Here's how the part is built. I have some questions about the finished solid (model axes, mm). A direction names the side the tool comes from. Round coordinates to 2 decimals unless told otherwise and drop trailing zeros. Write each loop counter-clockwise with the first axis right and the second up, starting at its lowest first coordinate (ties: lowest second). Pieces come first, ordered by that corner, then holes. Notation, with made-up numbers: (23.25, 12.25) -> (52.25, 12.25) arc R18 ccw to (52.25, 42.25) -> close; hole circle Ø7 at (-19, -6). An arc over 180 degrees is marked (long way). Put each result on its own line as item: value. Start each with the question number.
1) I want a section at A-A, the plane y = -15. List the corners of the cut face in (x, z) for me, then the cut area to 3 significant figures.
2) Which directions (+Z, -Z, +X, -X, +Y, -Y) give clear straight access to the entire face, cutting with the end or side of a thin tool? Please do faces 1 (the flat face through (-27.5, -15, -2)), 2 (the flat face through (-24, -15, -5)), 3 (the flat face through (24, -15, -5)).
3) We'd pull the mould along X, two halves only. Please class faces 4 (the flat face through (-23, -15, 0)), 5 (the cylindrical face through (0, -15, -15)), 6 (the cylindrical face through (-17.5, -14.9, -2.5)): released by +X, released by -X, zero draft, split by the parting line, or undercut.
4) Will these pins go through, and if not, where does the flat tip stop? P1, Ø6, axis at x = -8, z = -2, coming from the -Y side; P2, Ø4, axis at x = 19.5, y = -19, coming from the -Z side; P3, Ø4, axis at x = 8, y = -5, coming from the -Z side; P4, Ø1.5, axis at y = -21.5, z = -12.5, coming from the -X side.
5) If I drill on line 1 along Y through (x, z) = (-20, -3.65); line 2 along X through (y, z) = (-17, -4.25); line 3 along X through (y, z) = (-10.25, -4), over which ranges is the centre line in solid material (lowest first)? Write a range as [from, to].
6) I want a section at B-B, the plane x = 20. List the corners of the cut face in (y, z) for me, then the cut area to 3 significant figures.
7) I want a section at D-D, the plane z = -11.5. List the corners of the cut face in (x, y) for me, then the cut area to 3 significant figures.
8) I want a section at C-C, the plane z = -3.25. List the corners of the cut face in (x, y) for me, then the cut area to 3 significant figures.
from build123d import *

# Parameters (mm, degrees)
F1_DEPTH = 30
F3_D     = 5


with BuildPart() as f1:
    # F0 (on Front) → F1 (new body)
    with BuildSketch(Plane.XZ):
        with BuildLine():
            ThreePointArc((-14.1421356237, -5), (-14.7839783948, -2.5365296809), (-15, 0))
            Line((-15, 0), (-27.5, 0))
            Line((-27.5, 0), (-27.5, -5))
            Line((-27.5, -5), (-14.1421356237, -5))
        make_face()
        with BuildLine():
            ThreePointArc((-11.4564392374, -5), (-12.2363289116, -2.5538705461), (-12.5, 0))
            Line((-12.5, 0), (-15, 0))
            ThreePointArc((-15, 0), (-14.7839783948, -2.5365296809), (-14.1421356237, -5))
            Line((-14.1421356237, -5), (-11.4564392374, -5))
        make_face()
        with BuildLine():
            ThreePointArc((11.4564392374, -5), (0, -12.5), (-11.4564392374, -5))
            Line((-11.4564392374, -5), (-14.1421356237, -5))
            ThreePointArc((-14.1421356237, -5), (0, -15), (14.1421356237, -5))
            Line((14.1421356237, -5), (11.4564392374, -5))
        make_face()
        with BuildLine():
            ThreePointArc((12.5, 0), (12.2363289116, -2.5538705461), (11.4564392374, -5))
            Line((11.4564392374, -5), (14.1421356237, -5))
            ThreePointArc((14.1421356237, -5), (14.7839783948, -2.5365296809), (15, 0))
            Line((15, 0), (12.5, 0))
        make_face()
        with BuildLine():
            ThreePointArc((15, 0), (14.7839783948, -2.5365296809), (14.1421356237, -5))
            Line((14.1421356237, -5), (27.5, -5))
            Line((27.5, -5), (27.5, 0))
            Line((27.5, 0), (15, 0))
        make_face()
    extrude(amount=F1_DEPTH)

    # F3 (through all)
    with Locations(Plane.XY):
        with Locations((-20, -15), (20, -15)):
            Hole(F3_D / 2)


solid = f1.part
Findings:
1. outline: (-27.5, -5) -> (-22.5, -5) -> (-22.5, 0) -> (-27.5, 0) -> close; (-17.5, -5) -> (-14.14, -5) arc R15 ccw to (14.14, -5) -> (17.5, -5) -> (17.5, 0) -> (12.5, 0) arc R12.5 cw to (-12.5, 0) -> (-17.5, 0) -> close; (22.5, -5) -> (27.5, -5) -> (27.5, 0) -> (22.5, 0) -> close
1. area: 186 mm2
2. face 1: +Z, -Z, -X, +Y, -Y
2. face 2: -Z, -X, +Y, -Y
2. face 3: -Z, +X, +Y, -Y
3. face 4: zero draft
3. face 5: split by the parting line
3. face 6: undercut
4. P1: passes through
4. P2: stops at z = -5
4. P3: stops at z = -13.75
4. P4: stops at x = -9.32
5. line 1: y = [-30, -17.5], [-12.5, 0]
5. line 2: x = [-27.5, -21.5], [-18.5, -11.76], [11.76, 18.5], [21.5, 27.5]
5. line 3: x = [-27.5, -11.84], [11.84, 27.5]
6. outline: (-30, -5) -> (-17.5, -5) -> (-17.5, 0) -> (-30, 0) -> close; (-12.5, -5) -> (0, -5) -> (0, 0) -> (-12.5, 0) -> close
6. area: 125 mm2
7. outline: (-9.63, -30) -> (-4.9, -30) -> (-4.9, 0) -> (-9.63, 0) -> close; (4.9, -30) -> (9.63, -30) -> (9.63, 0) -> (4.9, 0) -> close
7. area: 284 mm2
8. outline: (-27.5, -30) -> (-12.07, -30) -> (-12.07, 0) -> (-27.5, 0) -> close; (12.07, -30) -> (27.5, -30) -> (27.5, 0) -> (12.07, 0) -> close; hole circle Ø5 at (-20, -15); hole circle Ø5 at (20, -15)
8. area: 887 mm2
